```python
from build123d import *

# Parameters (mm, degrees)
SKETCH1_W           = 310
SKETCH1_H           = 210
SKETCH1_R           = 3.5
BOSS_EXTRUDE1_DEPTH = 3
FILLET1_R           = 20
CUT_EXTRUDE2_DEPTH  = 10


with BuildPart() as part:
    # Sketch1 → Boss-Extrude1 (new body)
    with BuildSketch(Plane(origin=(0, 0, 0), x_dir=(1, 0, 0), z_dir=(0, 1, 0))):
        Rectangle(SKETCH1_W, SKETCH1_H)
        with Locations((-140, 90)):
            Circle(SKETCH1_R, mode=Mode.SUBTRACT)
        with Locations((140, 90)):
            Circle(SKETCH1_R, mode=Mode.SUBTRACT)
        with Locations((140, -90)):
            Circle(SKETCH1_R, mode=Mode.SUBTRACT)
        with Locations((-140, -90)):
            Circle(SKETCH1_R, mode=Mode.SUBTRACT)
        with Locations((102, -76)):
            Circle(SKETCH1_R, mode=Mode.SUBTRACT)
        with Locations((-37, -76)):
            Circle(SKETCH1_R, mode=Mode.SUBTRACT)
        with Locations((-64, 75)):
            Circle(SKETCH1_R, mode=Mode.SUBTRACT)
        with Locations((64, 75)):
            Circle(SKETCH1_R, mode=Mode.SUBTRACT)
        with Locations((-64, -5)):
            Circle(SKETCH1_R, mode=Mode.SUBTRACT)
        with Locations((64, -5)):
            Circle(SKETCH1_R, mode=Mode.SUBTRACT)
    extrude(amount=BOSS_EXTRUDE1_DEPTH)

    # Fillet1
    fillet1_edges = [part.edges().sort_by_distance(p)[0] for p in [
        (-155, 1.5, -105),
        (155, 1.5, -105),
        (155, 1.5, 105),
        (-155, 1.5, 105),
    ]]
    fillet(fillet1_edges, radius=FILLET1_R)

    # Sketch2 → Cut-Extrude2 (cut)
    with BuildSketch(Plane(origin=(0, 3, 0), x_dir=(1, 0, 0), z_dir=(0, 1, 0))):
        with BuildLine():
            Line((-107, 83), (-107, -3))
            ThreePointArc((-107, -3), (-106.414213562, -4.414213562), (-105, -5))
            Line((-105, -5), (-104.5, -5))
            ThreePointArc((-104.5, -5), (-103.085786438, -4.414213562), (-102.5, -3))
            Line((-102.5, -3), (-102.5, 83))
            ThreePointArc((-102.5, 83), (-103.085786438, 84.414213562), (-104.5, 85))
            Line((-104.5, 85), (-105, 85))
            ThreePointArc((-105, 85), (-106.414213562, 84.414213562), (-107, 83))
        make_face()
        with BuildLine():
            Line((-113, 85), (-112.5, 85))
            ThreePointArc((-112.5, 85), (-111.085786438, 84.414213562), (-110.5, 83))
            Line((-110.5, 83), (-110.5, -3))
            ThreePointArc((-110.5, -3), (-111.085786438, -4.414213562), (-112.5, -5))
            Line((-112.5, -5), (-113, -5))
            ThreePointArc((-113, -5), (-114.414213562, -4.414213562), (-115, -3))
            Line((-115, -3), (-115, 83))
            ThreePointArc((-115, 83), (-114.414213562, 84.414213562), (-113, 85))
        make_face()
        with BuildLine():
            Line((-99, 83), (-99, -3))
            ThreePointArc((-99, -3), (-98.414213562, -4.414213562), (-97, -5))
            Line((-97, -5), (-96.5, -5))
            ThreePointArc((-96.5, -5), (-95.085786438, -4.414213562), (-94.5, -3))
            Line((-94.5, -3), (-94.5, 83))
            ThreePointArc((-94.5, 83), (-95.085786438, 84.414213562), (-96.5, 85))
            Line((-96.5, 85), (-97, 85))
            ThreePointArc((-97, 85), (-98.414213562, 84.414213562), (-99, 83))
        make_face()
        with BuildLine():
            Line((-91, 83), (-91, -3))
            ThreePointArc((-91, -3), (-90.414213562, -4.414213562), (-89, -5))
            Line((-89, -5), (-88.5, -5))
            ThreePointArc((-88.5, -5), (-87.085786438, -4.414213562), (-86.5, -3))
            Line((-86.5, -3), (-86.5, 83))
            ThreePointArc((-86.5, 83), (-87.085786438, 84.414213562), (-88.5, 85))
            Line((-88.5, 85), (-89, 85))
            ThreePointArc((-89, 85), (-90.414213562, 84.414213562), (-91, 83))
        make_face()
        with BuildLine():
            Line((-83, 83), (-83, -3))
            ThreePointArc((-83, -3), (-82.414213562, -4.414213562), (-81, -5))
            Line((-81, -5), (-80.5, -5))
            ThreePointArc((-80.5, -5), (-79.085786438, -4.414213562), (-78.5, -3))
            Line((-78.5, -3), (-78.5, 83))
            ThreePointArc((-78.5, 83), (-79.085786438, 84.414213562), (-80.5, 85))
            Line((-80.5, 85), (-81, 85))
            ThreePointArc((-81, 85), (-82.414213562, 84.414213562), (-83, 83))
        make_face()
        with BuildLine():
            Line((5, 83), (5, -3))
            ThreePointArc((5, -3), (5.585786438, -4.414213562), (7, -5))
            Line((7, -5), (7.5, -5))
            ThreePointArc((7.5, -5), (8.914213562, -4.414213562), (9.5, -3))
            Line((9.5, -3), (9.5, 83))
            ThreePointArc((9.5, 83), (8.914213562, 84.414213562), (7.5, 85))
            Line((7.5, 85), (7, 85))
            ThreePointArc((7, 85), (5.585786438, 84.414213562), (5, 83))
        make_face()
        with BuildLine():
            Line((13, 83), (13, -3))
            ThreePointArc((13, -3), (13.585786438, -4.414213562), (15, -5))
            Line((15, -5), (15.5, -5))
            ThreePointArc((15.5, -5), (16.914213562, -4.414213562), (17.5, -3))
            Line((17.5, -3), (17.5, 83))
            ThreePointArc((17.5, 83), (16.914213562, 84.414213562), (15.5, 85))
            Line((15.5, 85), (15, 85))
            ThreePointArc((15, 85), (13.585786438, 84.414213562), (13, 83))
        make_face()
        with BuildLine():
            Line((21, 83), (21, -3))
            ThreePointArc((21, -3), (21.585786438, -4.414213562), (23, -5))
            Line((23, -5), (23.5, -5))
            ThreePointArc((23.5, -5), (24.914213562, -4.414213562), (25.5, -3))
            Line((25.5, -3), (25.5, 83))
            ThreePointArc((25.5, 83), (24.914213562, 84.414213562), (23.5, 85))
            Line((23.5, 85), (23, 85))
            ThreePointArc((23, 85), (21.585786438, 84.414213562), (21, 83))
        make_face()
        with BuildLine():
            Line((29, 83), (29, -3))
            ThreePointArc((29, -3), (29.585786438, -4.414213562), (31, -5))
            Line((31, -5), (31.5, -5))
            ThreePointArc((31.5, -5), (32.914213562, -4.414213562), (33.5, -3))
            Line((33.5, -3), (33.5, 83))
            ThreePointArc((33.5, 83), (32.914213562, 84.414213562), (31.5, 85))
            Line((31.5, 85), (31, 85))
            ThreePointArc((31, 85), (29.585786438, 84.414213562), (29, 83))
        make_face()
        with BuildLine():
            Line((37, 83), (37, -3))
            ThreePointArc((37, -3), (37.585786438, -4.414213562), (39, -5))
            Line((39, -5), (39.5, -5))
            ThreePointArc((39.5, -5), (40.914213562, -4.414213562), (41.5, -3))
            Line((41.5, -3), (41.5, 83))
            ThreePointArc((41.5, 83), (40.914213562, 84.414213562), (39.5, 85))
            Line((39.5, 85), (39, 85))
            ThreePointArc((39, 85), (37.585786438, 84.414213562), (37, 83))
        make_face()
        with BuildLine():
            Line((45, 83), (45, -3))
            ThreePointArc((45, -3), (45.585786438, -4.414213562), (47, -5))
            Line((47, -5), (47.5, -5))
            ThreePointArc((47.5, -5), (48.914213562, -4.414213562), (49.5, -3))
            Line((49.5, -3), (49.5, 83))
            ThreePointArc((49.5, 83), (48.914213562, 84.414213562), (47.5, 85))
            Line((47.5, 85), (47, 85))
            ThreePointArc((47, 85), (45.585786438, 84.414213562), (45, 83))
        make_face()
    extrude(amount=-CUT_EXTRUDE2_DEPTH, mode=Mode.SUBTRACT)


solid = part.part
```
The listing builds one solid part. Answer for the finished solid, in the listing's coordinates (mm). Coordinates: 2 decimals unless noted, no trailing zeros. Order: outer loops, then holes, each group sorted by start corner. A loop starts at its lowest first (then second) coordinate and runs counter-clockwise, first axis right, second up. Notation, with made-up numbers: M -16,51 L 33,51 A28 ccw 33,73 Z; hole C -5.5,34.5 d9. An arc over 180 degrees is marked long. Answer as a JSON object with one key per item and string values. Group by question number.
1. Section A-A on z = 76 is taken. Write down the section's boundary in (x, y), then the cut area to 3 significant figures.
2. Section C-C on z = -75 is taken. State how many separate pieces and enclosed holes the cut face has, then the cut area to 4 significant figures.
3. Section B-B on x = 64 is taken. Write down the section's boundary in (y, z), then the cut area to 3 significant figures.
4. Determine the mould class of faces 1 (the cylindrical face through (-149.297, 1.521, -98.986)), 2 (the cylindrical face through (148.986, 1.521, 99.297)), 3 (the cylindrical face through (-37.759, 1.479, 79.417)), 4 (the flat face through (-2, 3, -1)) for opening direction Z: released by +Z, released by -Z, zero draft, split by the parting line, or undercut.
5. Straight lines are drawn through the part: line 1 (Z direction, x = -64, y = 0.8); line 2 (Z direction, x = -96.5, y = 2.3); line 3 (X direction, y = 2.4, z = 74). For each, find the intervals that lie inside material, in ascending order.
6. A flat-ended cylindrical pin translates along its axis: P1, Ø4, axis at x = -140, z = 90, coming from the -Y side. Find the tip coordinate at first contact, or state that the pin passes through.
Values follow:
{
 "1": {"outline": "M -155,0 L -40.5,0 L -40.5,3 L -155,3 Z; M -33.5,0 L 98.5,0 L 98.5,3 L -33.5,3 Z; M 105.5,0 L 155,0 L 155,3 L 105.5,3 Z", "area": "888 mm2"},
 "2": {"separate pieces": "14", "enclosed holes": "0", "area": "739.5 mm2"},
 "3": {"outline": "M 0,-105 L 3,-105 L 3,-78.5 L 0,-78.5 Z; M 0,-71.5 L 3,-71.5 L 3,1.5 L 0,1.5 Z; M 0,8.5 L 3,8.5 L 3,105 L 0,105 Z", "area": "588 mm2"},
 "4": {"face 1": "released by -Z", "face 2": "released by +Z", "face 3": "undercut", "face 4": "zero draft"},
 "5": {"line 1": "-105 to -78.5, -71.5 to 1.5, 8.5 to 105", "line 2": "-105 to -85, 5 to 105", "line 3": "-155 to -39.87, -34.13 to 99.13, 104.87 to 155"},
 "6": {"P1": "through"}
}
